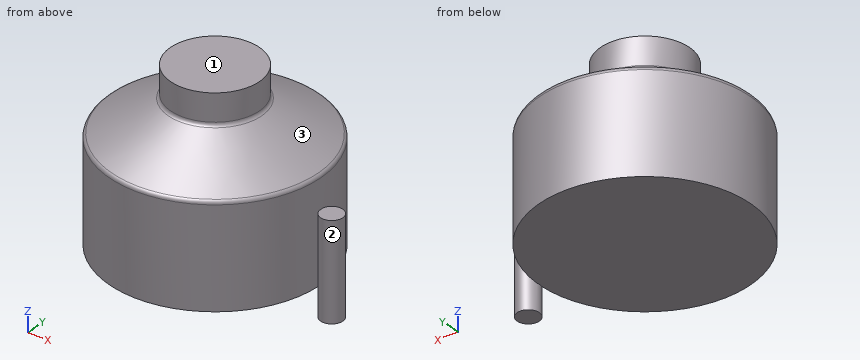
```python
from build123d import *

# Parameters (mm, degrees)
SKETCH3_W = 25
SKETCH3_H = 216.387840678


with BuildPart() as part:
    # Sketch2 → Revolve1 (revolve)
    with BuildSketch(Plane(origin=(0, 0, 0), x_dir=(1, 0, 0), z_dir=(0, 1, 0))):
        with BuildLine():
            Line((-232.5, -44.387840678), (-105, -118))
            ThreePointArc((-105, -118), (-101.339745962, -121.660254038), (-100, -126.660254038))
            Line((-100, -126.660254038), (-100, -188))
            Line((-100, -188), (0, -188))
            Line((0, -188), (0, 188))
            Line((0, 188), (-237.5, 188))
            Line((-237.5, 188), (-237.5, -35.72758664))
            ThreePointArc((-237.5, -35.72758664), (-236.160254038, -40.72758664), (-232.5, -44.387840678))
        make_face()
    revolve(axis=Axis((0, 0, -581.773938456), (0, 0, 1)))


with BuildPart() as body_2:
    # Sketch3 → Revolve2 (revolve)
    with BuildSketch(Plane(origin=(0, 0, 0), x_dir=(1, 0, 0), z_dir=(0, 1, 0))):
        with Locations((249, 138.806079661)):
            Rectangle(SKETCH3_W, SKETCH3_H)
    revolve(axis=Axis((261.5, 0, -182.650020504), (0, 0, 1)))

    # Combine3: union part
    add(part.part)


solid = body_2.part
```
Geometry check sheet. Reference: the model listing, model coordinates, mm. Face numbers are marked on the shaded views. Coordinates: 2 decimals unless noted, no trailing zeros. Order: outer loops, then holes, each group sorted by start corner. A loop starts at its lowest first (then second) coordinate and runs counter-clockwise, first axis right, second up. Notation, with made-up numbers: (-15.5, -13) - (5.5, -13) arc R31 ccw to (5.5, 14) - close; hole circle Ø1 at (17, -14.75). An arc over 180 degrees is marked (long way). Answer as a JSON object with one key per item and string values. Group by question number.
Item 1: Sectioned sample at A-A, the plane x = 0. Record the cut outline in (y, z), and give its area (3 significant figures).
Item 2: Sectioned sample at C-C, the plane z = 137. Record the cut outline in (x, y), and give its area (3 significant figures).
Item 3: Sectioned sample at D-D, the plane x = 261.5. Record the cut outline in (y, z).
Item 4: Depth check by flat-ended pin: pin 1 Ø1.5 at (x, y) = (-22.5, 95.5) entering from -Z; pin 2 Ø4 at (x, y) = (-95, -128.5) entering from +Z; pin 3 Ø1.5 at (y, z) = (-55.5, -132) entering from +X. Enter the tip coordinate at first touch or a pass-through.
Item 5: Sectioned sample at B-B, the plane y = 0. Record the cut outline in (x, z).
Item 6: Draft check along X on the marked faces 1, 2 and 3. Enter one of: +X half, -X half, draft (parallel to the pull), parting line (faces both ways), or undercut.
Item 7: Scan lines: probe 1 along Z at (x, y) = (-38, -64.5); probe 2 along Z at (x, y) = (-135, 28); probe 3 along X at (y, z) = (203, -129.5). Record each from-to range of solid material in increasing order.
Resolved:
{
 "1": {"outline": "(-237.5, -188) - (237.5, -188) - (237.5, 35.73) arc R10 ccw to (232.5, 44.39) - (105, 118) arc R10 cw to (100, 126.66) - (100, 188) - (-100, 188) - (-100, 126.66) arc R10 cw to (-105, 118) - (-232.5, 44.39) arc R10 ccw to (-237.5, 35.73) - close", "area": "149,000 mm^2"},
 "2": {"outline": "circle Ø200 at (0, 0)", "area": "31,400 mm^2"},
 "3": {"outline": "(-25, -247) - (25, -247) - (25, -30.61) - (-25, -30.61) - close"},
 "4": {"pin 1": "z = -188", "pin 2": "z = 87.51", "pin 3": "x = 231.1"},
 "5": {"outline": "(-237.5, -188) - (236.5, -188) - (236.5, -247) - (286.5, -247) - (286.5, -30.61) - (237.5, -30.61) - (237.5, 35.73) arc R10 ccw to (232.5, 44.39) - (105, 118) arc R10 cw to (100, 126.66) - (100, 188) - (-100, 188) - (-100, 126.66) arc R10 cw to (-105, 118) - (-232.5, 44.39) arc R10 ccw to (-237.5, 35.73) - close"},
 "6": {"face 1": "draft", "face 2": "undercut", "face 3": "parting line"},
 "7": {"probe 1": "-188 to 188", "probe 2": "-188 to 99.02", "probe 3": "-123.28 to 123.28"}
}
